Geometry check sheet. Reference: the model listing, model coordinates, mm. Coordinates: 2 decimals unless noted, no trailing zeros. Loops run counter-clockwise (first coordinate to the right, second up) from the corner with the lowest first, then second, coordinate; pieces in that order, holes last.
from build123d import *

# Parameters (mm, degrees)
SKETCH2_R               = 22.5
BOSS_EXTRUDE1_DEPTH     = 3.175
SKETCH3_R               = 3.25755
SKETCH3_R_2             = 2.15
CUT_EXTRUDE1_DEPTH      = 1
CUT_EXTRUDE1_DEPTH_BACK = 7.35
SKETCH4_R               = 2.25
CUT_EXTRUDE2_DEPTH      = 1
CUT_EXTRUDE2_DEPTH_BACK = 7.35


with BuildPart() as part:
    # Sketch2 → Boss-Extrude1 (new body, symmetric)
    with BuildSketch(Plane.XY):
        Polygon((-34.925, 0), (34.925, 0), (34.925, 81.7), (34.925, 114.2), (34.925, 129.2), (-34.925, 129.2), (-34.925, 114.2), (-34.925, 81.7), align=None)
        with Locations((0, 81.7)):
            Circle(SKETCH2_R, mode=Mode.SUBTRACT)
    extrude(amount=BOSS_EXTRUDE1_DEPTH, both=True)

    # Sketch3 → Cut-Extrude1 (cut, two sides)
    with BuildSketch(Plane.XY.offset(3.175)) as cut_extrude1_sk:
        with Locations((-25.425, 12.7)):
            Circle(SKETCH3_R)
        with Locations((25.425, 12.7)):
            Circle(SKETCH3_R)
        with Locations((22.425, 122.7)):
            Circle(SKETCH3_R_2)
    extrude(amount=CUT_EXTRUDE1_DEPTH, mode=Mode.SUBTRACT)
    extrude(cut_extrude1_sk.sketch, amount=-CUT_EXTRUDE1_DEPTH_BACK, mode=Mode.SUBTRACT)

    # Sketch4 → Cut-Extrude2 (cut, two sides)
    with BuildSketch(Plane(origin=(0, 0, -3.175), x_dir=(-1, 0, 0), z_dir=(0, 0, -1))) as cut_extrude2_sk:
        with Locations((-28, 107.7)):
            Circle(SKETCH4_R)
        with Locations((28, 107.7)):
            Circle(SKETCH4_R)
        with Locations((-28, 55.7)):
            Circle(SKETCH4_R)
        with Locations((28, 55.7)):
            Circle(SKETCH4_R)
    extrude(amount=CUT_EXTRUDE2_DEPTH, mode=Mode.SUBTRACT)
    extrude(cut_extrude2_sk.sketch, amount=-CUT_EXTRUDE2_DEPTH_BACK, mode=Mode.SUBTRACT)


solid = part.part
1) Section check C-C on z = 1.75. Count the separate pieces of the cut face and the enclosed holes in it, and give its area (3 significant figures).
Data:
separate pieces: 1
enclosed holes: 8
area: 7,290 mm2
2) Section check B-B on x = -18. Record the cut outline in (y, z) (3 decimals), and give its area (3 significant figures).
Data:
outline: (0, -3.175) - (68.2, -3.175) - (68.2, 3.175) - (0, 3.175) - close; (95.2, -3.175) - (129.2, -3.175) - (129.2, 3.175) - (95.2, 3.175) - close
area: 649 mm2
3) Mould release check, pull along X, two halves, no side actions. Record for faces 1 (the flat face through (-34.925, 66, 0)), 2 (the flat face through (0, 129.2, 0)), 3 (the cylindrical face through (28.29, 109.93, -0.04)), 4 (the cylindrical face through (-26.13, 9.52, 0.04)): +X half, -X half, draft (parallel to the pull), parting line (faces both ways), or undercut.
Data:
face 1: -X half
face 2: draft
face 3: undercut
face 4: undercut
4) Material ranges on probe 1 along Y at (x, z) = (0, 1.25); probe 2 along Y at (x, z) = (27, -1); probe 3 along Y at (x, z) = (28, -0.5), recorded low to high.
Data:
probe 1: y = 0 to 59.2, 104.2 to 129.2
probe 2: y = 0 to 9.85, 15.55 to 53.68, 57.72 to 105.68, 109.72 to 129.2
probe 3: y = 0 to 10.7, 14.7 to 53.45, 57.95 to 105.45, 109.95 to 129.2
5) Section check A-A on y = 107.7. Record the cut outline in (x, z) (3 decimals).
Data:
outline: (-34.925, -3.175) - (-30.25, -3.175) - (-30.25, 3.175) - (-34.925, 3.175) - close; (-25.75, -3.175) - (25.75, -3.175) - (25.75, 3.175) - (-25.75, 3.175) - close; (30.25, -3.175) - (34.925, -3.175) - (34.925, 3.175) - (30.25, 3.175) - close
6) Section check D-D on y = 81.7. Record the cut outline in (x, z) (3 decimals), and give its area (3 significant figures).
Data:
outline: (-34.925, -3.175) - (-22.5, -3.175) - (-22.5, 3.175) - (-34.925, 3.175) - close; (22.5, -3.175) - (34.925, -3.175) - (34.925, 3.175) - (22.5, 3.175) - close
area: 158 mm2
7) Depth check by flat-ended pin: pin 1 (6 mm diameter, centred on x = 28, y = 55.7, fed in from -Z) (3 decimals); pin 2 (3.5 mm diameter, centred on x = -28, y = 107.7, fed in from +Z). Enter the tip coordinate at first touch or a pass-through.
Data:
pin 1: stops at z = -3.175
pin 2: passes through
